Print and shaded views of the part. All mm, measured from the part's lowest x, y and z. Coordinates: 2 decimals unless noted, no trailing zeros. Loops run counter-clockwise (first coordinate to the right, second up) from the corner with the lowest first, then second, coordinate; pieces in that order, holes last.
1) Pin check, flat tip, straight feed: pin 1 Ø1.8 at (x, z) = (3, 6) entering from +Y. Stop position of the tip, or through.
2) Saw through at B-B, the plane z = 6. Write the cut outline in (x, y).
3) Saw through at C-C, the plane y = 0.7. Write the cut outline in (x, z).
4) Saw through at A-A, the plane x = 7. Write the cut outline in (y, z).
5) Wall check: line 1 along X through (y, z) = (1.4, 3); line 2 along X through (y, z) = (1.65, 6); line 3 along Z through (x, y) = (14, 0.7). Give the ranges that are in metal, low to high.
6) Saw through at D-D, the plane x = 2.75. Write the cut outline in (y, z), and give its area (3 significant figures).
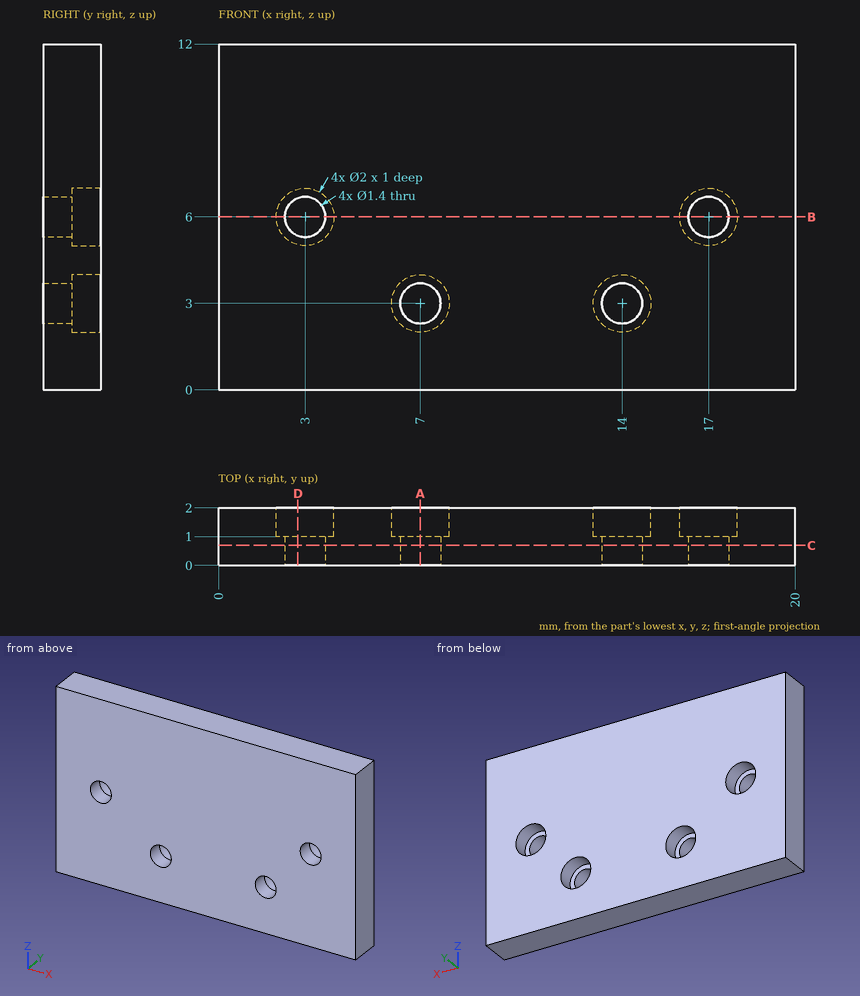
Data:
1. pin 1: stops at y = 1
2. outline: (0, 0) - (2.3, 0) - (2.3, 1) - (2, 1) - (2, 2) - (0, 2) - close; (3.7, 0) - (16.3, 0) - (16.3, 1) - (16, 1) - (16, 2) - (4, 2) - (4, 1) - (3.7, 1) - close; (17.7, 0) - (20, 0) - (20, 2) - (18, 2) - (18, 1) - (17.7, 1) - close
3. outline: (0, 0) - (20, 0) - (20, 12) - (0, 12) - close; hole circle Ø1.4 at (3, 6); hole circle Ø1.4 at (7, 3); hole circle Ø1.4 at (14, 3); hole circle Ø1.4 at (17, 6)
4. outline: (0, 0) - (2, 0) - (2, 2) - (1, 2) - (1, 2.3) - (0, 2.3) - close; (0, 3.7) - (1, 3.7) - (1, 4) - (2, 4) - (2, 12) - (0, 12) - close
5. line 1: x = 0 to 6, 8 to 13, 15 to 20
5. line 2: x = 0 to 2, 4 to 16, 18 to 20
5. line 3: z = 0 to 2.3, 3.7 to 12
6. outline: (0, 0) - (2, 0) - (2, 5.03) - (1, 5.03) - (1, 5.35) - (0, 5.35) - close; (0, 6.65) - (1, 6.65) - (1, 6.97) - (2, 6.97) - (2, 12) - (0, 12) - close
6. area: 20.8 mm2
